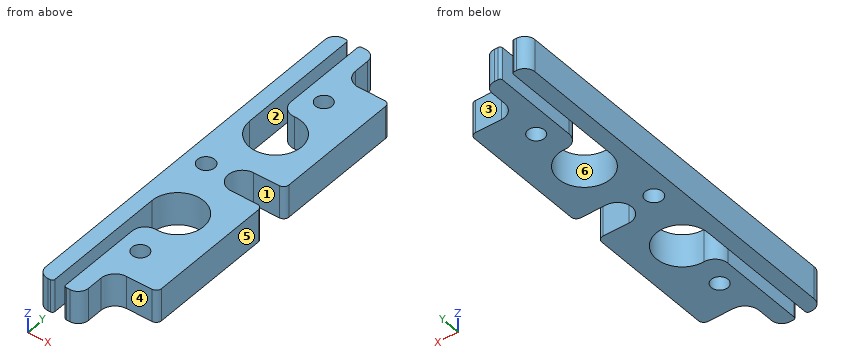
Autodesk Inventor part; units mm, degrees
ref_plane "YZ Plane" through (0, 0, 0) normal (1, 0, 0) x (0, 1, 0)
ref_plane "XZ Plane" through (0, 0, 0) normal (0, 1, 0) x (-1, 0, 0)
ref_plane "XY Plane" through (0, 0, 0) normal (0, 0, 1) x (1, 0, 0)
sketch "Sketch1" plane through (0, 0, 0) normal (0, 0, 1) x (1, 0, 0)
  line L0 (8.5, -36.236) -> (-8.5, -36.236)
  line L1 (-8.5, -36.236) -> (-8.5, 36.236)
  line L2 (-8.5, 36.236) -> (8.5, 36.236)
  line L3 (8.5, 36.236) -> (8.5, -36.236)
  line L4 (8.5, -36.236) -> (-8.5, 36.236) construction
  line L5 (-8.5, -36.236) -> (8.5, 36.236) construction
  line L6 (8.5, 0) -> (2.5, 0) construction
  line L7 (8.5, 2.75) -> (2.5, 2.75)
  line L8 (2.5, -2.75) -> (8.5, -2.75)
  arc A0 (8.5, -2.75) -> (8.5, 2.75) centre (8.5, 0) ccw
  arc A1 (2.5, 2.75) -> (2.5, -2.75) centre (2.5, 0) ccw
  line L9 (8.5, 36.236) -> (-0.25, 36.236)
  line L10 (-0.25, 36.236) -> (-0.25, 31.236)
  line L11 (2.5, 28.486) -> (8.5, 28.486)
  line L12 (8.5, 28.486) -> (8.5, 36.236)
  line L13 (8.5, -36.236) -> (-0.25, -36.236)
  line L14 (-0.25, -36.236) -> (-0.25, -31.236)
  line L15 (2.5, -28.486) -> (8.5, -28.486)
  line L16 (8.5, -28.486) -> (8.5, -36.236)
  arc A2 (2.5, -28.486) -> (-0.25, -31.236) centre (2.5, -31.236) ccw
  arc A3 (-0.25, 31.236) -> (2.5, 28.486) centre (2.5, 31.236) ccw
  line L17 (0.5, 22.5) -> (0.5, -22.5) construction
  line L18 (-5.55, 36.236) -> (-3.45, 36.236)
  line L19 (-3.45, 36.236) -> (-3.45, -36.236)
  line L20 (-3.45, -36.236) -> (-5.55, -36.236)
  line L21 (-5.55, -36.236) -> (-5.55, 36.236)
  line L22 (-8.5, 36.236) -> (-0.25, 36.236)
  circle A4 centre (-0.55, 12) radius 3.5
  circle A5 centre (-0.55, 12) radius 5
  circle A6 centre (-0.95, 19.4893) radius 2.5
  circle A7 centre (-4.5, 0) radius 4 construction
  point P0 (0, 0)
  point P1 (5.5, 0)
  point P2 (0.5, 0)
  point P3 (-8.5, 0)
  point P4 (-0.25, -36.236)
  point P5 (8.5, -28.486)
  point P6 (-0.25, 36.236)
  point P7 (-0.8167, 16.9929)
  point P8 (-3.45, 19.4893)
  point P9 (-3.45, 36.236)
  point P10 (-5.55, 36.236)
  point P11 (-5.55, 12)
  dimension "d0" = 17
  dimension "d1" = 72.472
  dimension "d3" = 5.5
  dimension "d4" = 11
  dimension "d6" = 5
  dimension "d7" = 5
  dimension "d8" = 45
  dimension "d9" = 9
  dimension "d22" = 2.1
  dimension "d24" = 7
  dimension "d25" = 1.5
  dimension "d26" = 5
  dimension "d27" = 12
  dimension "d29" = 8
  dimension "d40" = 2.95
extrude "Extrusion1" add sketch "Sketch1" along normal blind 6.35 contours L0 L19 A5 A6 L2 L10 A3 L11 L3 L7 A1 L8 L15 A2 L14 | L0 L21 A5 L19 | L0 L1 L2 L21 | A5 L19 A4 | L19 A4 A5 | L21 L2 L19 A5 | A4 L19 | L19 A4 | L19 A6 A5 | A6
fillet "Fillet1" radius 2 2 edges at (-8.5, -36.236, 3.175) (-8.5, 36.236, 3.175)
fillet "Fillet2" radius 2 2 edges at (-0.25, -36.236, 3.175) (-0.25, 36.236, 3.175)
fillet "Fillet3" radius 1 4 edges at (8.5, -28.486, 3.175) (8.5, -2.75, 3.175) (8.5, 2.75, 3.175) (8.5, 28.486, 3.175)
hole "Hole1" at (0.5, 22.5, 0) at (0.5, -22.5, 0) direction (0, 0, 1) diameter 3.2 end through all
hole "Hole2" at (-4.5, 0, 0) direction (0, 0, 1) diameter 3.3 end through all
extrude "Extrusion2" cut sketch "Sketch1" along normal blind 6.35 contours A5 L19 A4 | L19 A4 A5 | L21 L2 L19 A5 | A4 L19 | L19 A4 | L19 A6 A5
mirror "Mirror1" about plane through (0, 0, 0) normal (0, 1, 0) of "Extrusion2"
fillet "Fillet4" radius 0.5 4 edges at (-5.55, 36.236, 3.175) (-3.45, 36.236, 3.175) (-3.45, -36.236, 3.175) (-5.55, -36.236, 3.175)
equation "\"d7\" = d6"
properties part number "Gantry Belt Clamp" material "Aluminum 6061"
Build history of the part. All positions in model axes, mm. Face numbers are marked on the shaded views. A direction names the side the tool comes from. Coordinates: 2 decimals unless noted, no trailing zeros. Order: outer loops, then holes, each group sorted by start corner. A loop starts at its lowest first (then second) coordinate and runs counter-clockwise, first axis right, second up. Notation, with made-up numbers: (-3, 29.5) -> (32, 29.5) arc R13 ccw to (32, 52.5) -> close; hole circle Ø7 at (54.25, 37.5). An arc over 180 degrees is marked (long way). Answer in a Markdown table with one row per item. Add a question column.
Q1. Band-saw the part on A-A, the plane y = -22.5. List the corners of the cut face in (x, z).
Q2. Band-saw the part on C-C, the plane x = 0.5. List the corners of the cut face in (y, z), then the cut area to 3 significant figures.
Q3. Wall check: line 1 along X through (y, z) = (-22.5, 4.25); line 2 along X through (y, z) = (-32.5, 4.5); line 3 along X through (y, z) = (-12, 5). Give the ranges that are in metal, low to high. Write a range as [from, to].
Q4. Band-saw the part on D-D, the plane y = 9.5. List the corners of the cut face in (x, z), then the cut area to 3 significant figures.
Q5. Drop flat-ended pins along their axis: pin 1 (1.5 mm diameter, centred on x = 5.5, z = 4.5, fed in from +Y); pin 2 (3.5 mm diameter, centred on y = -33.5, z = 4.5, fed in from +X); pin 3 (1.5 mm diameter, centred on x = 5, z = 3, fed in from -Y). Give the stop position or say it passes through.
Q6. Which spindle directions (+Z, -Z, +X, -X, +Y, -Y) get a long thin tool onto all of the face, cutting with end or side? Do the marked faces 1, 2 and 3. Say none if no direction does.
Q7. Mould opens along Y. For the marked faces 4, 5 and 6 say: +Y half, -Y half, draft (parallel to the pull), parting line (faces both ways), or undercut.
Q8. Band-saw the part on B-B, the plane x = 5.5. List the corners of the cut face in (y, z).
Answers follow:
| question | item | result |
|---|---|---|
| 1 | outline | (-8.5, 0) -> (-5.55, 0) -> (-5.55, 6.35) -> (-8.5, 6.35) -> close; (-3.45, 0) -> (-1.1, 0) -> (-1.1, 6.35) -> (-3.45, 6.35) -> close; (2.1, 0) -> (8.5, 0) -> (8.5, 6.35) -> (2.1, 6.35) -> close |
| 2 | outline | (-29.35, 0) -> (-24.1, 0) -> (-24.1, 6.35) -> (-29.35, 6.35) -> close; (-20.9, 0) -> (-16.89, 0) -> (-16.89, 6.35) -> (-20.9, 6.35) -> close; (-7.11, 0) -> (-1.89, 0) -> (-1.89, 6.35) -> (-7.11, 6.35) -> close; (1.89, 0) -> (7.11, 0) -> (7.11, 6.35) -> (1.89, 6.35) -> close; (16.89, 0) -> (20.9, 0) -> (20.9, 6.35) -> (16.89, 6.35) -> close; (24.1, 0) -> (29.35, 0) -> (29.35, 6.35) -> (24.1, 6.35) -> close |
| 2 | area | 184 mm^2 |
| 3 | line 1 | [-8.5, -5.55], [-3.45, -1.1], [2.1, 8.5] |
| 3 | line 2 | [-8.5, -5.55], [-3.45, -0.25] |
| 3 | line 3 | [-8.5, -5.55], [4.45, 8.5] |
| 4 | outline | (-8.5, 0) -> (-4.88, 0) -> (-4.88, 6.35) -> (-8.5, 6.35) -> close; (3.78, 0) -> (8.5, 0) -> (8.5, 6.35) -> (3.78, 6.35) -> close |
| 4 | area | 53.0 mm^2 |
| 5 | pin 1 | y = 28.49 |
| 5 | pin 2 | x = -0.25 |
| 5 | pin 3 | y = -28.49 |
| 6 | face 1 | +Z, -Z, +X |
| 6 | face 2 | +Z, -Z, +Y |
| 6 | face 3 | +Z, -Z, +X, +Y |
| 7 | face 4 | -Y half |
| 7 | face 5 | draft |
| 7 | face 6 | undercut |
| 8 | outline | (-28.49, 0) -> (-2.75, 0) -> (-2.75, 6.35) -> (-28.49, 6.35) -> close; (2.75, 0) -> (28.49, 0) -> (28.49, 6.35) -> (2.75, 6.35) -> close |
